Design review of the part built by this model. Coordinates are the model's own, in mm. Coordinates: 2 decimals unless noted, no trailing zeros. Write each loop counter-clockwise with the first axis right and the second up, starting at its lowest first coordinate (ties: lowest second). Pieces come first, ordered by that corner, then holes.
Q1. To check wall thickness, follow probe 1 along Z at (x, y) = (0, -4.25); probe 2 along Z at (x, y) = (0, -4.75); probe 3 along X at (y, z) = (-7.25, -2.5). State the ranges of each line that lie inside material, in increasing order.
Q2. Add section B-B, the plane y = -0.75. Give the boundary of the cut face in (x, z), plus the area to 3 significant figures.
Q3. Clearance check with flat-ended pins moving along their axes: pin 1 Ø1 at (x, z) = (-5.5, -0.5) entering from -Y; pin 2 Ø1.5 at (x, y) = (5.5, 5) entering from +Z; pin 3 Ø10 at (x, y) = (5.5, 3.5) entering from -Z. State where each tip first meets the part, or that it passes through.
Q4. Add section A-A, the plane z = 0. Give the boundary of the cut face in (x, y) (3 decimals), plus the area to 3 significant figures.
Q5. Add section C-C, the plane x = 0. Give the boundary of the cut face in (y, z) (3 decimals).
Q6. Add section D-D, the plane y = 3.25. Give the boundary of the cut face in (x, z).
from build123d import *

# Parameters (mm, degrees)
F3_R     = 3.6917022886
F4_DEPTH = 25.4


with BuildPart() as f2:
    # F0 (on Front) → F2 (revolve)
    with BuildSketch(Plane.XZ):
        with BuildLine():
            Line((0, -9.525), (0, 9.525))
            ThreePointArc((0, 9.525), (-9.525, 0), (0, -9.525))
        make_face()
    revolve(axis=Axis((0, 0, 0), (0, 0, 1)))


with BuildPart() as f4:
    # F3 (on Front) → F4 (new body)
    with BuildSketch(Plane.XZ):
        Circle(F3_R)
    extrude(amount=F4_DEPTH)


with BuildPart() as f2_1:
    add(f2.part)

    # F5: cut F4
    add(f4.part, mode=Mode.SUBTRACT)


solid = f2_1.part
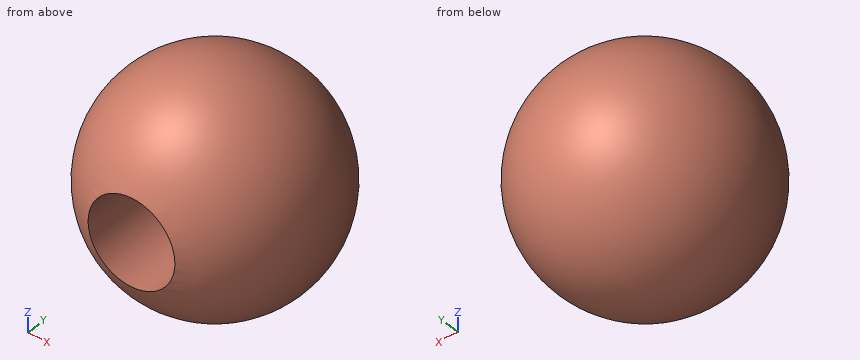
Here are the results:
1. probe 1: z = -8.52 to -3.69, 3.69 to 8.52
1. probe 2: z = -8.26 to -3.69, 3.69 to 8.26
1. probe 3: x = -5.65 to -2.72, 2.72 to 5.65
2. outline: circle Ø18.99 at (0, 0); hole circle Ø7.38 at (0, 0)
2. area: 240 mm2
3. pin 1: stops at y = -8.09
3. pin 2: stops at z = 6.79
3. pin 3: stops at z = -9.4
4. outline: (-3.692, -8.78) - (-3.692, 0) - (3.692, 0) - (3.692, -8.78) arc R9.525 ccw (long way) to start
4. area: 216 mm2
5. outline: (-8.78, -3.692) arc R9.525 ccw (long way) to (-8.78, 3.692) - (0, 3.692) - (0, -3.692) - close
6. outline: circle Ø17.91 at (0, 0)
